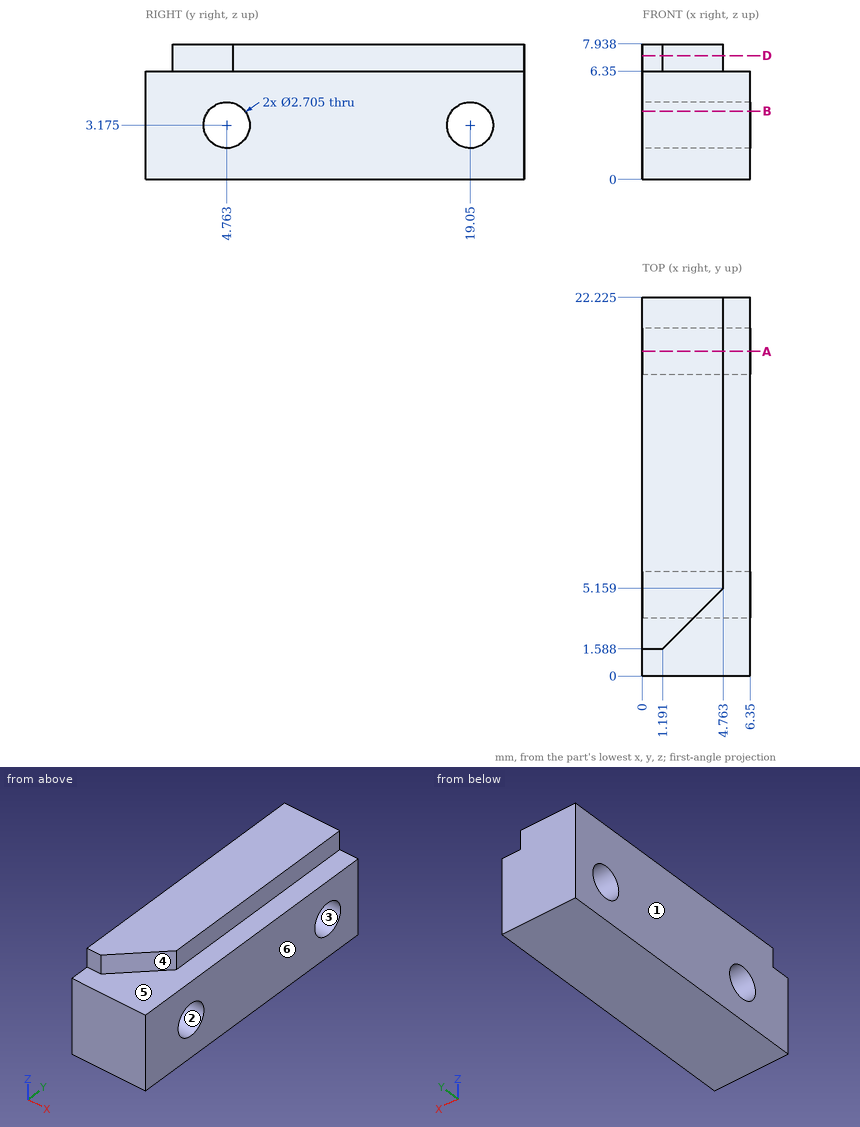
The figure shows three views and two pictorial views of one solid part (mm, origin at its lowest corner). Answer the questions. A direction names the side the tool comes from. Round coordinates to 2 decimals unless told otherwise and drop trailing zeros. Write each loop counter-clockwise with the first axis right and the second up, starting at its lowest first coordinate (ties: lowest second). Pieces come first, ordered by that corner, then holes. Notation, with made-up numbers: M 1,-1.5 L 13,-1.5 A19 ccw 13,9.5 Z; hole C 29.5,11.5 d5. An arc over 180 degrees is marked long. Write each question's results on one line, items separated by ' | '. Start each with the question number.
(1) The part is cut by section A-A, the plane y = 19.05. Write down the section's boundary in (x, z), and give its area (3 significant figures).
(2) Find the intervals of material crossed by line 1 (Z direction, x = 1.5, y = 19.05); line 2 (Y direction, x = 2.25, z = 2.5) (1 decimal); line 3 (Y direction, x = 4, z = 4.25) (1 decimal), in increasing order.
(3) For the marked faces 5 and 6, determine the directions among +Z, -Z, +X, -X, +Y, -Y from which every point of the face is accessible in a straight line to the end or side of a thin tool.
(4) Determine the mould class of the marked faces 1, 2, 3 and 4 for opening direction Y: +Y half, -Y half, draft (parallel to the pull), parting line (faces both ways), or undercut.
(5) Each of these flat-tipped pins is pushed along its axis until it touches: P1, Ø4.5, axis at y = 4.76, z = 3.18, coming from the +X side; P2, Ø2, axis at y = 19.05, z = 3.175, coming from the +X side; P3, Ø1, axis at x = 0.5, z = 7, coming from the -Y side; P4, Ø1, axis at x = 5, y = 2.5, coming from the +Z side. Where does it stop, or does it pass through?
(6) The part is cut by section B-B, the plane z = 4. Give the number of separate pieces and of enclosed holes in the cut face, and give its area (3 significant figures).
(7) The part is cut by section D-D, the plane z = 7.25. Write down the section's boundary in (x, y) (1 decimal).
Worked answers:
1) outline: M 0,0 L 6.35,0 L 6.35,1.82 L 0,1.82 Z; M 0,4.53 L 6.35,4.53 L 6.35,6.35 L 4.76,6.35 L 4.76,7.94 L 0,7.94 Z | area: 30.7 mm²
2) line 1: z = 0 to 1.82, 4.53 to 7.94 | line 2: y = 0 to 3.6, 5.9 to 17.9, 20.2 to 22.2 | line 3: y = 0 to 3.9, 5.6 to 18.2, 19.9 to 22.2
3) face 5: +Z, +X, -Y | face 6: +Z, -Z, +X, +Y, -Y
4) face 1: draft | face 2: undercut | face 3: undercut | face 4: -Y half
5) P1: stops at x = 6.35 | P2: passes through | P3: stops at y = 1.59 | P4: stops at z = 6.35
6) separate pieces: 3 | enclosed holes: 0 | area: 114 mm²
7) outline: M 0,1.6 L 1.2,1.6 L 4.8,5.2 L 4.8,22.2 L 0,22.2 Z
